```python
from build123d import *

# Parameters (mm, degrees)
SKETCH1_R           = 1.651
BOSS_EXTRUDE1_DEPTH = 3.175


with BuildPart() as part:
    # Sketch1 → Boss-Extrude1 (new body)
    with BuildSketch(Plane(origin=(0, 0, 0), x_dir=(1, 0, 0), z_dir=(0, 1, 0))):
        Polygon((38.1, -12.7), (25.4, -12.7), (25.4, 0), (6.35, 0), (6.35, -12.7), (25.4, -31.75), (38.1, -31.75), align=None)
        with Locations((32.54375, -19.05)):
            Circle(SKETCH1_R, mode=Mode.SUBTRACT)
        with Locations((32.54375, -25.4)):
            Circle(SKETCH1_R, mode=Mode.SUBTRACT)
        with Locations((12.7, -5.55625)):
            Circle(SKETCH1_R, mode=Mode.SUBTRACT)
        with Locations((19.05, -5.55625)):
            Circle(SKETCH1_R, mode=Mode.SUBTRACT)
    extrude(amount=BOSS_EXTRUDE1_DEPTH)


solid = part.part
```
Source: CAD feature listing. Evaluate the final solid. Frame: model axes, mm. A direction names the side the tool comes from. Coordinates: 2 decimals unless noted, no trailing zeros. Order: outer loops, then holes, each group sorted by start corner. A loop starts at its lowest first (then second) coordinate and runs counter-clockwise, first axis right, second up. Notation, with made-up numbers: M -39.5,51.25 L 10.5,51.25 A16 ccw 10.5,66.25 Z; hole C 51,-2.5 d5. An arc over 180 degrees is marked long. Write each question's results on one line, items separated by ' | '. Start each with the question number.
1) Section query B-B (x = 19.05). Return the cut outline in (y, z) (3 decimals), plus the area to 3 significant figures.
2) Draft query along X for faces 3 (the face through (6.35, 2, 6)), 4 (the face through (22, 3.175, 16)), 5 (the face through (31.33, 1.57, 24.28)). Return one class per face: released by +X, released by -X, zero draft, split by the parting line, or undercut.
3) Line query: line 1 (Z direction, x = 19.05, y = 1.5); line 2 (Z direction, x = 26.5, y = 3); line 3 (X direction, y = 1.8, z = 25.4). Output: solid intervals per line, ascending. Write a range as from..to.
4) Contact query for flat-ended pins moving along their axis: pin 1 Ø1.6 at (x, y) = (29.5, 1.5) entering from -Z; pin 2 Ø2.5 at (x, z) = (32.54, 19.05) entering from +Y. Output: stop coordinate, or through.
5) Access query for faces 1 (the face through (16, 2, 0)), 2 (the face through (25.4, 2, 6)). Directions: +Z, -Z, +X, -X, +Y, -Y. A direction counts if a zero-diameter tool reaches every point of the face in a straight line with its end or side. Return the directions, or none.
6) Section query C-C (x = 33.5). Return the cut outline in (y, z) (3 decimals), plus the area to 3 significant figures.
7) Section query D-D (z = 6.5). Return the cut outline in (x, y) (3 decimals), plus the area to 3 significant figures.
8) Section query A-A (z = 19.05). Return the cut outline in (x, y) (3 decimals).
Answers:
1) outline: M 0,0 L 3.175,0 L 3.175,3.905 L 0,3.905 Z; M 0,7.207 L 3.175,7.207 L 3.175,25.4 L 0,25.4 Z | area: 70.2 mm^2
2) face 3: released by -X | face 4: zero draft | face 5: undercut
3) line 1: z = 0..3.91, 7.21..25.4 | line 2: z = 12.7..31.75 | line 3: x = 19.05..30.89, 34.19..38.1
4) pin 1: stops at z = 12.7 | pin 2: passes through
5) face 1: -Z, +X, -X, +Y, -Y | face 2: -Z, +X, +Y, -Y
6) outline: M 0,12.7 L 3.175,12.7 L 3.175,17.704 L 0,17.704 Z; M 0,20.396 L 3.175,20.396 L 3.175,24.054 L 0,24.054 Z; M 0,26.746 L 3.175,26.746 L 3.175,31.75 L 0,31.75 Z | area: 43.4 mm^2
7) outline: M 6.35,0 L 11.345,0 L 11.345,3.175 L 6.35,3.175 Z; M 14.055,0 L 17.695,0 L 17.695,3.175 L 14.055,3.175 Z; M 20.405,0 L 25.4,0 L 25.4,3.175 L 20.405,3.175 Z | area: 43.3 mm^2
8) outline: M 12.7,0 L 30.893,0 L 30.893,3.175 L 12.7,3.175 Z; M 34.195,0 L 38.1,0 L 38.1,3.175 L 34.195,3.175 Z
